```python
from build123d import *

# Parameters (mm, degrees)
SKETCH5_W               = 82.5
SKETCH5_H               = 35.530981805
BOSS_EXTRUDE1_DEPTH     = 3
SKETCH8_R               = 53.75957742
SKETCH8_R_2             = 38
CUT_EXTRUDE1_DEPTH      = 13
SKETCH7_W               = 25.1
SKETCH7_H               = 23.6
CUT_EXTRUDE2_DEPTH      = 2
SKETCH10_W              = 6
SKETCH10_H              = 6
BOSS_EXTRUDE2_DEPTH     = 15
CUT_EXTRUDE3_DEPTH      = 12
CUT_EXTRUDE4_DEPTH      = 12
CUT_EXTRUDE5_DEPTH      = 17
CUT_EXTRUDE5_DEPTH_BACK = 12
SKETCH15_R              = 1.5
SKETCH16_R              = 1.2
CUT_EXTRUDE6_DEPTH      = 10


with BuildPart() as part:
    # Sketch5 → Boss-Extrude1 (new body)
    with BuildSketch(Plane.XY):
        with Locations((41.25, 4.834509098)):
            Rectangle(SKETCH5_W, SKETCH5_H)
    extrude(amount=BOSS_EXTRUDE1_DEPTH)

    # Sketch8 → Cut-Extrude1 (cut)
    with BuildSketch(Plane.XY.offset(3)):
        with Locations((41.25, 11.3)):
            Circle(SKETCH8_R)
        with Locations((41.25, 11.3)):
            Circle(SKETCH8_R_2, mode=Mode.SUBTRACT)
    extrude(amount=-CUT_EXTRUDE1_DEPTH, mode=Mode.SUBTRACT)

    # Sketch7 → Cut-Extrude2 (cut)
    with BuildSketch(Plane.XY.offset(3)):
        with Locations((20.303816898, 16.8)):
            Rectangle(SKETCH7_W, SKETCH7_H)
    extrude(amount=-CUT_EXTRUDE2_DEPTH, mode=Mode.SUBTRACT)

    # Sketch10 → Boss-Extrude2 (add)
    with BuildSketch(Plane(origin=(0, 0, 0), x_dir=(-1, 0, 0), z_dir=(0, 0, -1))):
        with Locations((-59.301708923, 1.6)):
            Rectangle(SKETCH10_W, SKETCH10_H)
        with Locations((-59.301708923, 19.6)):
            Rectangle(SKETCH10_W, SKETCH10_H)
    extrude(amount=BOSS_EXTRUDE2_DEPTH)

    # Sketch11 → Cut-Extrude3 (cut)
    with BuildSketch(Plane.ZY.offset(-56.301708923)):
        with BuildLine():
            Line((-15.673682817, 18.188265047), (-15.673682817, 24.450923395))
            Line((-15.673682817, 24.450923395), (0, 24.450923395))
            Line((0, 24.450923395), (0, 22.6))
            add(Edge.make_bspline(
                [(0, 22.6), (-3.159886635, 22.462578072), (-7.547752793, 18.690290822), (-13.247203151, 18.200972407), (-15.673682817, 18.188265047)],
                knots=[0, 0, 0, 0, 0.549888978, 1, 1, 1, 1], degree=3))
        make_face()
        with BuildLine():
            Line((-10.484624341, 16.6), (-10.708289412, 12.015073246))
            Line((-10.708289412, 12.015073246), (0, 12.015073246))
            Line((0, 12.015073246), (0, 20.424934677))
            add(Edge.make_bspline(
                [(0, 20.424934677), (-1.83740901, 20.191851474), (-5.266921055, 18.665051954), (-8.555682053, 16.881899659), (-10.484624341, 16.6)],
                knots=[0, 0, 0, 0, 0.489527902, 1, 1, 1, 1], degree=3))
        make_face()
        with BuildLine():
            Line((0, 9.184926754), (0, 0.775065323))
            add(Edge.make_bspline(
                [(0, 0.775065323), (-1.83740901, 1.008148526), (-5.266921055, 2.534948046), (-8.555682053, 4.318100341), (-10.484624341, 4.6)],
                knots=[0, 0, 0, 0, 0.489527902, 1, 1, 1, 1], degree=3))
            Line((-10.484624341, 4.6), (-10.708289412, 9.184926754))
            Line((-10.708289412, 9.184926754), (0, 9.184926754))
        make_face()
        with BuildLine():
            Line((0, -3.250923395), (0, -1.4))
            add(Edge.make_bspline(
                [(0, -1.4), (-3.159886635, -1.262578072), (-7.547752793, 2.509709178), (-13.247203151, 2.999027593), (-15.673682817, 3.011734953)],
                knots=[0, 0, 0, 0, 0.549888978, 1, 1, 1, 1], degree=3))
            Line((-15.673682817, 3.011734953), (-15.673682817, -3.250923395))
            Line((-15.673682817, -3.250923395), (0, -3.250923395))
        make_face()
    extrude(amount=-CUT_EXTRUDE3_DEPTH, mode=Mode.SUBTRACT)

    # Sketch14 → Cut-Extrude4 (cut)
    with BuildSketch(Plane(origin=(0, 0, 0), x_dir=(-1, 0, 0), z_dir=(0, 0, -1))):
        with BuildLine():
            Line((-71.618289014, 16.6), (-51.598213122, 16.6))
            ThreePointArc((-51.598213122, 16.6), (-45.598213122, 10.6), (-51.598213122, 4.6))
            Line((-51.598213122, 4.6), (-71.618289014, 4.6))
            ThreePointArc((-71.618289014, 4.6), (-77.618289014, 10.6), (-71.618289014, 16.6))
        make_face()
    extrude(amount=-CUT_EXTRUDE4_DEPTH, mode=Mode.SUBTRACT)

    # Sketch15 → Cut-Extrude5 (cut, two sides: drawn at the far end of the back side and taken through both)
    with BuildSketch(Plane(origin=(0, 16.6, 0), x_dir=(-1, 0, 0), z_dir=(0, -1, 0)).offset(-CUT_EXTRUDE5_DEPTH_BACK)):
        with Locations(Location((-59.266135992, 12.650675834, 0), (0, 0, 90))):
            Circle(SKETCH15_R)
    extrude(amount=CUT_EXTRUDE5_DEPTH + CUT_EXTRUDE5_DEPTH_BACK, mode=Mode.SUBTRACT)

    # Sketch16 → Cut-Extrude6 (cut)
    with BuildSketch(Plane.XY.offset(1)):
        with BuildLine():
            ThreePointArc((12.053816898, 13.5), (10.853816898, 14.7), (9.653816898, 13.5))
            Line((9.653816898, 13.5), (10.853816898, 13.5))
            Line((10.853816898, 13.5), (10.853816898, 12.3))
            ThreePointArc((10.853816898, 12.3), (11.702345036, 12.651471863), (12.053816898, 13.5))
        make_face()
        with BuildLine():
            Line((10.853816898, 13.5), (9.653816898, 13.5))
            ThreePointArc((9.653816898, 13.5), (10.005288761, 12.651471863), (10.853816898, 12.3))
            Line((10.853816898, 12.3), (10.853816898, 13.5))
        make_face()
        with Locations((29.753816898, 13.5)):
            Circle(SKETCH16_R)
    extrude(amount=-CUT_EXTRUDE6_DEPTH, mode=Mode.SUBTRACT)


solid = part.part
```
For this review, take the finished solid that the model builds, in its own axes (mm). A direction names the side the tool comes from. Round coordinates to 2 decimals unless told otherwise and drop trailing zeros. Write each loop counter-clockwise with the first axis right and the second up, starting at its lowest first coordinate (ties: lowest second). Pieces come first, ordered by that corner, then holes.
1) Machinability: for faces 4 (the face through (61, 16.6, -13)), 5 (the face through (59.332, 3.638, -11.152)), 6 (the face through (62.302, 2, -7)), 7 (the face through (20, 14, 1)), 8 (the face through (45.6, 10.7, 1.5)), which of the approach directions +Z, -Z, +X, -X, +Y, -Y give a long, thin tool a straight path to every point of the face, cutting with its end or side? Answer none if there is none.
Answer below:
face 4: +Z, -Z, +X, -X
face 5: +Y, -Y
face 6: -Z, +X, +Y, -Y
face 7: +Z, +Y
face 8: +Z, -Z
2) Take a section at B-B on x = 50.5. Give the boundary of the cut face in (y, z).
Answer below:
outline: (-12.93, 0) - (4.7, 0) - (4.7, 3) - (-12.93, 3) - close; (16.5, 0) - (22.6, 0) - (22.6, 3) - (16.5, 3) - close
3) Take a section at C-C on z = -12. State how many separate pieces and enclosed holes the cut face has, then the cut area to 3 significant figures.
Answer below:
separate pieces: 4
enclosed holes: 0
area: 12.0 mm2
4) Take a section at D-D on x = 32. Give the boundary of the cut face in (y, z), then the cut area to 3 significant figures.
Answer below:
outline: (-12.93, 0) - (22.6, 0) - (22.6, 1) - (5, 1) - (5, 3) - (-12.93, 3) - close
area: 71.4 mm2
5) For line 1 along Z through (x, y) = (7.5, 7); line 2 along Z through (x, y) = (21, 16); line 3 along X through (y, z) = (1, -6.25), list the stretches that pass through material, from the lowest coordinate up.
Answer below:
line 1: z = 0 to 3
line 2: z = 0 to 1
line 3: x = 56.3 to 62.3
6) Mouldability with a two-part tool opening along X and no side actions: class faces 1 (the face through (3.918, 4.205, 1.521)), 2 (the face through (41, 5, 0)), 3 (the face through (32.854, 14, 2)) as +X half, -X half, draft (parallel to the pull), parting line (faces both ways), or undercut.
Answer below:
face 1: -X half
face 2: draft
face 3: undercut
7) Take a section at A-A on y = 10.6. Give the boundary of the cut face in (x, z).
Answer below:
outline: (3.26, 0) - (45.6, 0) - (45.6, 3) - (32.85, 3) - (32.85, 1) - (7.75, 1) - (7.75, 3) - (3.26, 3) - close; (77.62, 0) - (79.24, 0) - (79.24, 3) - (77.62, 3) - close
8) Insertion check: pin 1 Ø2 at (x, z) = (15, 2.5) entering from +Y; pin 2 Ø10 at (x, y) = (58.5, 11) entering from -Z; pin 3 Ø2 at (y, z) = (17, 2.5) entering from -X; pin 4 Ø5 at (x, z) = (59.27, -12.65) entering from +Y. Each pin has a flat end and moves straight along its axis. Give the tip position at first contact, or say it passes through.
Answer below:
pin 1: stops at y = 5
pin 2: passes through
pin 3: stops at x = 3.54
pin 4: stops at y = 18.76
